Read the model definition and answer for the solid it produces. Units are mm, in the model's axes. A direction names the side the tool comes from. Coordinates: 2 decimals unless noted, no trailing zeros. Loops run counter-clockwise (first coordinate to the right, second up) from the corner with the lowest first, then second, coordinate; pieces in that order, holes last.
from build123d import *

# Parameters (mm, degrees)
SKETCH1_W           = 165
SKETCH1_H           = 150
BOSS_EXTRUDE1_DEPTH = 30
SKETCH2_W           = 135
SKETCH2_H           = 135
SKETCH2_W_2         = 127
SKETCH2_H_2         = 126
CUT_EXTRUDE1_DEPTH  = 9
CUT_EXTRUDE2_DEPTH  = 2
SKETCH4_R           = 2.5
CUT_EXTRUDE3_DEPTH  = 11
SKETCH5_W           = 210
SKETCH5_H           = 210
BOSS_EXTRUDE2_DEPTH = 5
FILLET1_R           = 10
SKETCH6_R           = 4.4
CUT_EXTRUDE4_DEPTH  = 211.535032714
CHAMFER1_SIZE       = 5
CUT_EXTRUDE5_DEPTH  = 9
FILLET2_R           = 2
SKETCH8_R           = 1.9
CUT_EXTRUDE6_DEPTH  = 25
SKETCH10_R          = 3.25
CUT_EXTRUDE8_DEPTH  = 7.5
SKETCH9_R           = 2.5
CUT_EXTRUDE7_DEPTH  = 10


with BuildPart() as part:
    # Sketch1 → Boss-Extrude1 (new body)
    with BuildSketch(Plane(origin=(0, 0, 0), x_dir=(1, 0, 0), z_dir=(0, 1, 0))):
        Rectangle(SKETCH1_W, SKETCH1_H)
    extrude(amount=BOSS_EXTRUDE1_DEPTH)

    # Sketch2 → Cut-Extrude1 (cut)
    with BuildSketch(Plane(origin=(0, 30, 0), x_dir=(1, 0, 0), z_dir=(0, 1, 0))):
        with Locations((0, -0.5)):
            Rectangle(SKETCH2_W, SKETCH2_H)
        Rectangle(SKETCH2_W_2, SKETCH2_H_2, mode=Mode.SUBTRACT)
    extrude(amount=-CUT_EXTRUDE1_DEPTH, mode=Mode.SUBTRACT)

    # Sketch3 → Cut-Extrude2 (cut)
    with BuildSketch(Plane(origin=(0, 30, 0), x_dir=(1, 0, 0), z_dir=(0, 1, 0))):
        Polygon((75.5, -10), (72.5, -10), (72.5, 0), (69, 0), (74, 7.5), (79, 0), (75.5, 0), align=None)
    cut_extrude2 = extrude(amount=-CUT_EXTRUDE2_DEPTH, mode=Mode.SUBTRACT)

    # Mirror1: Cut-Extrude2 across plane
    add(cut_extrude2.mirror(Plane(origin=(0, 0, 0), x_dir=(0, 0, 1), z_dir=(1, 0, 0))), mode=Mode.SUBTRACT)

    # Sketch4 → Cut-Extrude3 (cut)
    with BuildSketch(Plane.XY.offset(75)):
        with Locations((72.5, 25)):
            Circle(SKETCH4_R)
        with Locations((-72.5, 25)):
            Circle(SKETCH4_R)
    extrude(amount=-CUT_EXTRUDE3_DEPTH, mode=Mode.SUBTRACT)

    # Sketch5 → Boss-Extrude2 (add)
    with BuildSketch(Plane.XZ):
        Rectangle(SKETCH5_W, SKETCH5_H)
    extrude(amount=-BOSS_EXTRUDE2_DEPTH)

    # Fillet1
    fillet1_edges = [part.edges().sort_by_distance(p)[0] for p in [
        (105, 2.5, 105),
        (105, 2.5, -105),
        (-105, 2.5, -105),
        (-105, 2.5, 105),
    ]]
    fillet(fillet1_edges, radius=FILLET1_R)

    # Sketch6 → Cut-Extrude4 (cut, through all)
    with BuildSketch(Plane.XY.offset(75)):
        with Locations((-57.5, 12)):
            Circle(SKETCH6_R)
        with Locations((57.5, 12)):
            Circle(SKETCH6_R)
    extrude(amount=-CUT_EXTRUDE4_DEPTH, mode=Mode.SUBTRACT)

    # Chamfer1
    chamfer1_edges = [part.edges().sort_by_distance(p)[0] for p in [
        (63.5, 30, 0),
        (0, 30, 63),
        (-63.5, 30, 0),
        (0, 30, -63),
    ]]
    chamfer(chamfer1_edges, length=CHAMFER1_SIZE)

    # Sketch7 → Cut-Extrude5 (cut)
    with BuildSketch(Plane(origin=(0, 30, 0), x_dir=(1, 0, 0), z_dir=(0, 1, 0))):
        with BuildLine():
            Line((-67.5, 65.5), (-67.5, 67))
            Line((-67.5, 67), (-66, 67))
            ThreePointArc((-66, 67), (-68.560660172, 68.060660172), (-67.5, 65.5))
        make_face()
        with BuildLine():
            Line((66, 67), (67.5, 67))
            Line((67.5, 67), (67.5, 65.5))
            ThreePointArc((67.5, 65.5), (68.560660172, 68.060660172), (66, 67))
        make_face()
        with BuildLine():
            Line((66, -68), (67.5, -68))
            Line((67.5, -68), (67.5, -66.5))
            ThreePointArc((67.5, -66.5), (68.560660172, -69.060660172), (66, -68))
        make_face()
        with BuildLine():
            Line((-67.5, -66.5), (-67.5, -68))
            Line((-67.5, -68), (-66, -68))
            ThreePointArc((-66, -68), (-68.560660172, -69.060660172), (-67.5, -66.5))
        make_face()
    extrude(amount=-CUT_EXTRUDE5_DEPTH, mode=Mode.SUBTRACT)

    # Fillet2
    fillet2_edges = [part.edges().sort_by_distance(p)[0] for p in [
        (-67.5, 25.5, 66.5),
        (-66, 25.5, 68),
        (66, 25.5, 68),
        (67.5, 25.5, 66.5),
        (67.5, 25.5, -65.5),
        (66, 25.5, -67),
        (-67.5, 25.5, -65.5),
        (-66, 25.5, -67),
        (63.5, 23, 63),
        (-63.5, 23, 63),
        (-63.5, 23, -63),
        (63.5, 23, -63),
    ]]
    fillet(fillet2_edges, radius=FILLET2_R)

    # Sketch8 → Cut-Extrude6 (cut)
    with BuildSketch(Plane(origin=(82.5, 0, 0), x_dir=(0, 0, -1), z_dir=(1, 0, 0))):
        with Locations((-60, 12)):
            Circle(SKETCH8_R)
    cut_extrude6 = extrude(amount=-CUT_EXTRUDE6_DEPTH, mode=Mode.SUBTRACT)

    # Sketch10 → Cut-Extrude8 (cut)
    with BuildSketch(Plane(origin=(82.5, 0, 0), x_dir=(0, 0, -1), z_dir=(1, 0, 0))):
        with Locations((-60, 12)):
            Circle(SKETCH10_R)
    cut_extrude8 = extrude(amount=-CUT_EXTRUDE8_DEPTH, mode=Mode.SUBTRACT)

    # Mirror2: Cut-Extrude6, Cut-Extrude8 across plane
    add(cut_extrude6.mirror(Plane(origin=(0, 0, 0), x_dir=(0, 0, 1), z_dir=(1, 0, 0))), mode=Mode.SUBTRACT)
    add(cut_extrude8.mirror(Plane(origin=(0, 0, 0), x_dir=(0, 0, 1), z_dir=(1, 0, 0))), mode=Mode.SUBTRACT)

    # Sketch9 → Cut-Extrude7 (cut)
    with BuildSketch(Plane(origin=(-82.5, 0, 0), x_dir=(0, 0, -1), z_dir=(1, 0, 0))):
        with Locations((-50, 17.5)):
            Circle(SKETCH9_R)
        with Locations((50, 17.5)):
            Circle(SKETCH9_R)
    extrude(amount=CUT_EXTRUDE7_DEPTH, mode=Mode.SUBTRACT)


solid = part.part
Item 1: Determine the mould class of faces 4 (the face through (-72.5, 18, 50)), 5 (the face through (-1, 17, -75)), 6 (the face through (-1, 17, 75)), 7 (the face through (-82.5, 17, 1)) for opening direction Z: released by +Z, released by -Z, zero draft, split by the parting line, or undercut.
Numbers:
face 4: undercut
face 5: released by -Z
face 6: released by +Z
face 7: zero draft
Item 2: Find the intervals of material crossed by line 1 along Y through (x, z) = (-76, -50); line 2 along Y through (x, z) = (-78.5, 60); line 3 along X through (y, z) = (26, -59), in increasing order.
Numbers:
line 1: y = 0 to 15, 20 to 30
line 2: y = 0 to 8.75, 15.25 to 30
line 3: x = -82.5 to -67.5, -62.5 to 62.5, 67.5 to 82.5
Item 3: A cutting plane is placed at A-A on z = 12.5. Determine the outline of the cut face in (x, y), then the cut area to 3 significant figures.
Numbers:
outline: (-105, 0) - (105, 0) - (105, 5) - (82.5, 5) - (82.5, 30) - (67.5, 30) - (67.5, 21) - (63.5, 21) - (63.5, 25) - (58.5, 30) - (-58.5, 30) - (-63.5, 25) - (-63.5, 21) - (-67.5, 21) - (-67.5, 30) - (-82.5, 30) - (-82.5, 5) - (-105, 5) - close; hole circle Ø8.8 at (-57.5, 12); hole circle Ø8.8 at (57.5, 12)
area: 4,960 mm2
Item 4: Which of the six approach directions +Z, -Z, +X, -X, +Y, -Y give full straight-line access (tool end or side, diameter ignored) to faces 1 (the face through (-77.57, 18.251, -52.385)), 2 (the face through (-1, 26, 68)), 3 (the face through (78.802, 12.143, 63.247))?
Numbers:
face 1: -X
face 2: +Y
face 3: +X
Item 5: A cutting plane is placed at B-B on x = 2.5. Determine the outline of the cut face in (y, z).
Numbers:
outline: (0, -105) - (5, -105) - (5, -75) - (30, -75) - (30, -67) - (21, -67) - (21, -63) - (25, -63) - (30, -58) - (30, 58) - (25, 63) - (21, 63) - (21, 68) - (30, 68) - (30, 75) - (5, 75) - (5, 105) - (0, 105) - close
Item 6: Given pin 1 (1 mm diameter, centred on x = -71, y = 29.5, fed in from -Z); pin 2 (2 mm diameter, centred on y = 23.5, z = 46, fed in from +X); pin 3 (6 mm diameter, centred on x = -14.5, z = -23.5, fed in from -Y); pin 4 (1.5 mm diameter, centred on x = 26.5, y = 17.5, fed in from +Z), each flat-ended and moving along its own axis, determine where each tip first touches the part or whether it passes through.
Numbers:
pin 1: stops at z = -75
pin 2: stops at x = 82.5
pin 3: stops at y = 0
pin 4: stops at z = 75
Item 7: A cutting plane is placed at D-D on x = 85. Determine the outline of the cut face in (y, z), then the cut area to 3 significant figures.
Numbers:
outline: (0, -105) - (5, -105) - (5, 105) - (0, 105) - close
area: 1,050 mm2
Item 8: A cutting plane is placed at C-C on z = 50. Determine the outline of the cut face in (x, y).
Numbers:
outline: (-105, 0) - (105, 0) - (105, 5) - (82.5, 5) - (82.5, 30) - (67.5, 30) - (67.5, 21) - (63.5, 21) - (63.5, 25) - (58.5, 30) - (-58.5, 30) - (-63.5, 25) - (-63.5, 21) - (-67.5, 21) - (-67.5, 30) - (-82.5, 30) - (-82.5, 20) - (-72.5, 20) - (-72.5, 15) - (-82.5, 15) - (-82.5, 5) - (-105, 5) - close; hole circle Ø8.8 at (-57.5, 12); hole circle Ø8.8 at (57.5, 12)
